```python
from build123d import *

# Parameters (mm, degrees)
SKETCH1_R           = 1.75
SKETCH1_W           = 55.7
SKETCH1_H           = 26
SKETCH1_W_2         = 31.5
SKETCH1_H_2         = 20.5
SKETCH1_W_3         = 27.4
SKETCH1_H_3         = 16.5
BOSS_EXTRUDE1_DEPTH = 2
SKETCH1_3_W         = 31.5
SKETCH1_3_H         = 20.5
SKETCH1_3_W_2       = 27.4
SKETCH1_3_H_2       = 16.5
BOSS_EXTRUDE2_DEPTH = 1
FILLET1_R           = 1
CHAMFER1_SIZE       = 1.9


with BuildPart() as part:
    # Sketch1 → Boss-Extrude1 (new body)
    # profile 1 of 3: a face of its own
    with BuildSketch(Plane(origin=(0, 0, 0), x_dir=(1, 0, 0), z_dir=(0, 1, 0))):
        with BuildLine():
            Line((-39.25, 22), (28.45, 22))
            ThreePointArc((28.45, 22), (31.278427125, 20.828427125), (32.45, 18))
            Line((32.45, 18), (32.45, -18))
            ThreePointArc((32.45, -18), (31.278427125, -20.828427125), (28.45, -22))
            Line((28.45, -22), (-39.25, -22))
            ThreePointArc((-39.25, -22), (-42.078427125, -20.828427125), (-43.25, -18))
            Line((-43.25, -18), (-43.25, 18))
            ThreePointArc((-43.25, 18), (-42.078427125, 20.828427125), (-39.25, 22))
        make_face()
        with Locations(Location((-38.25, -18, 0), (0, 0, 270))):
            Circle(SKETCH1_R, mode=Mode.SUBTRACT)
        with Locations(Location((27.45, 18, 0), (0, 0, 270))):
            Circle(SKETCH1_R, mode=Mode.SUBTRACT)
        with Locations(Location((-38.25, 18, 0), (0, 0, 270))):
            Circle(SKETCH1_R, mode=Mode.SUBTRACT)
        with Locations(Location((-5.4, 18, 0), (0, 0, 270))):
            Circle(SKETCH1_R, mode=Mode.SUBTRACT)
        with Locations(Location((27.45, -18, 0), (0, 0, 270))):
            Circle(SKETCH1_R, mode=Mode.SUBTRACT)
        with Locations(Location((-5.4, -18, 0), (0, 0, 270))):
            Circle(SKETCH1_R, mode=Mode.SUBTRACT)
        with Locations((-5.4, 0)):
            Rectangle(SKETCH1_W, SKETCH1_H, mode=Mode.SUBTRACT)
    # profile 2 of 3: a face of its own
    with BuildSketch(Plane(origin=(0, 0, 0), x_dir=(1, 0, 0), z_dir=(0, 1, 0))):
        with Locations((-5.4, 0)):
            Rectangle(SKETCH1_W, SKETCH1_H)
        Rectangle(SKETCH1_W_2, SKETCH1_H_2, mode=Mode.SUBTRACT)
    # profile 3 of 3: a face of its own
    with BuildSketch(Plane(origin=(0, 0, 0), x_dir=(1, 0, 0), z_dir=(0, 1, 0))):
        Rectangle(SKETCH1_W_2, SKETCH1_H_2)
        Rectangle(SKETCH1_W_3, SKETCH1_H_3, mode=Mode.SUBTRACT)
    extrude(amount=BOSS_EXTRUDE1_DEPTH)

    # Sketch1_3 → Boss-Extrude2 (add)
    with BuildSketch(Plane(origin=(0, 0, 0), x_dir=(1, 0, 0), z_dir=(0, 1, 0))):
        Rectangle(SKETCH1_3_W, SKETCH1_3_H)
        Rectangle(SKETCH1_3_W_2, SKETCH1_3_H_2, mode=Mode.SUBTRACT)
    extrude(amount=BOSS_EXTRUDE2_DEPTH)

    # Fillet1
    fillet1_edges = [part.edges().sort_by_distance(p)[0] for p in [
        (-5.4, 2, -22),
        (-42.078427125, 2, -20.828427125),
        (-43.25, 2, 0),
        (-42.078427125, 2, 20.828427125),
        (-5.4, 2, 22),
        (31.278427125, 2, 20.828427125),
        (32.45, 2, 0),
        (31.278427125, 2, -20.828427125),
    ]]
    fillet(fillet1_edges, radius=FILLET1_R)

    # Chamfer1
    chamfer1_edges = [part.edges().sort_by_distance(p)[0] for p in [
        (13.7, 2, 0),
        (0, 2, 8.25),
        (-13.7, 2, 0),
        (0, 2, -8.25),
    ]]
    chamfer(chamfer1_edges, length=CHAMFER1_SIZE)


solid = part.part
```
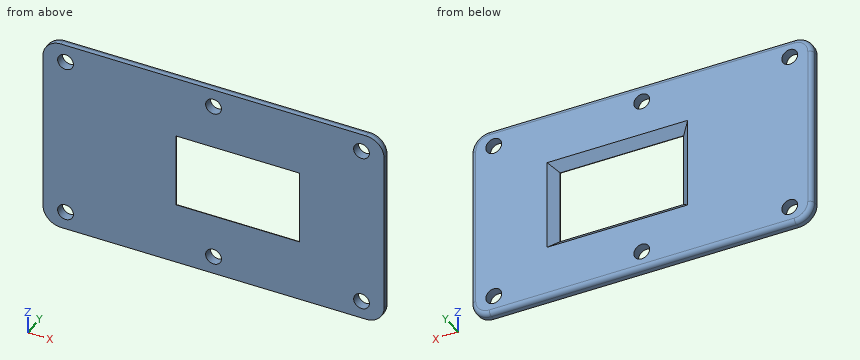
CAD build for the part. Positions are in the model's coordinates, mm. Coordinates: 2 decimals unless noted, no trailing zeros. Write each loop counter-clockwise with the first axis right and the second up, starting at its lowest first coordinate (ties: lowest second). Pieces come first, ordered by that corner, then holes. Notation, with made-up numbers: (66.25, 36) -> (115.25, 36) arc R27 cw to (115.25, 60) -> close; hole circle Ø8 at (23.5, 88). An arc over 180 degrees is marked (long way). Use CSV: the item, a comma, the result in double quotes. Start each with the question number.
Item 1: Band-saw the part on A-A, the plane y = 0.45. Write the cut outline in (x, z), plus the area to 3 significant figures.
Item 2: Wall check: probe 1 along X at (y, z) = (0.9, 18); probe 2 along Z at (x, y) = (-37, 0.3); probe 3 along X at (y, z) = (0.85, 19). Give the ranges that are in metal, low to high.
Item 3: Band-saw the part on B-B, the plane x = -5.4. Write the cut outline in (y, z).
Item 4: Band-saw the part on C-C, the plane x = -38.25. Write the cut outline in (y, z), plus the area to 3 significant figures.
Response values:
1,outline,"(-43.25, -18) arc R4 ccw to (-39.25, -22) -> (28.45, -22) arc R4 ccw to (32.45, -18) -> (32.45, 18) arc R4 ccw to (28.45, 22) -> (-39.25, 22) arc R4 ccw to (-43.25, 18) -> close; hole circle Ø3.5 at (-38.25, -18); hole circle Ø3.5 at (-38.25, 18); hole (-14.05, -8.6) -> (14.05, -8.6) -> (14.05, 8.6) -> (-14.05, 8.6) -> close; hole circle Ø3.5 at (-5.4, -18); hole circle Ø3.5 at (-5.4, 18); hole circle Ø3.5 at (27.45, -18); hole circle Ø3.5 at (27.45, 18)"
1,area,"2,780 mm2"
2,probe 1,"x = -43.25 to -40, -36.5 to -7.15, -3.65 to 25.7, 29.2 to 32.45"
2,probe 2,"z = -22 to -19.22, -16.78 to 16.78, 19.22 to 22"
2,probe 3,"x = -43.12 to -39.69, -36.81 to -6.84, -3.96 to 26.01, 28.89 to 32.32"
3,outline,"(0, -22) -> (1, -22) arc R1 ccw to (2, -21) -> (2, -19.75) -> (0, -19.75) -> close; (0, -16.25) -> (2, -16.25) -> (2, -10.15) -> (0.1, -8.25) -> (0, -8.25) -> close; (0, 8.25) -> (0.1, 8.25) -> (2, 10.15) -> (2, 16.25) -> (0, 16.25) -> close; (0, 19.75) -> (2, 19.75) -> (2, 21) arc R1 ccw to (1, 22) -> (0, 22) -> close"
4,outline,"(0, -22) -> (1, -22) arc R1 ccw to (2, -21) -> (2, -19.75) -> (0, -19.75) -> close; (0, -16.25) -> (2, -16.25) -> (2, 16.25) -> (0, 16.25) -> close; (0, 19.75) -> (2, 19.75) -> (2, 21) arc R1 ccw to (1, 22) -> (0, 22) -> close"
4,area,"73.6 mm2"
